Source: three-view drawing plus pictorial views. Frame: mm from the lowest corner of the part. Give positions to 0.01 mm unless a question says otherwise; leave off trailing zeros. Write each loop counter-clockwise with the first axis right and the second up, starting at its lowest first coordinate (ties: lowest second). Pieces come first, ordered by that corner, then holes.
Q1. Cut plane C-C on x = 216. Return the cut outline in (y, z), plus the area to 3 significant figures.
Q2. Cut plane B-B on y = 136.5. Return the cut outline in (x, z), plus the area to 3 significant figures.
Q3. Draft query along Y for the marked faces 1 and 2. Return one class per face: pulls with the +Y half, pulls with the -Y half, needs draft (parallel to the pull), parting line crosses it, or undercut.
Q4. Cut plane D-D on y = 228. Return the cut outline in (x, z), plus the area to 3 significant figures.
Q5. Cut plane A-A on z = 136.5. Return the cut outline in (x, y).
Q6. Pin query (flat end, axial travel): pin 1 (2 mm diameter, centred on x = 117, z = 224.5, fed in from +Y); pin 2 (8 mm diameter, centred on x = 319.5, z = 57, fed in from -Y); pin 3 (8 mm diameter, centred on x = 178.5, z = 287, fed in from +Y). Return the tip coordinate at first contact, or that it passes through.
Q7. Line query: L1, parallel to Z at x = 233, y = 136; L2, parallel to Y at x = 162, z = 143; L3, parallel to Y at x = 216, z = 288.5. Output: solid intervals per line, ascending.
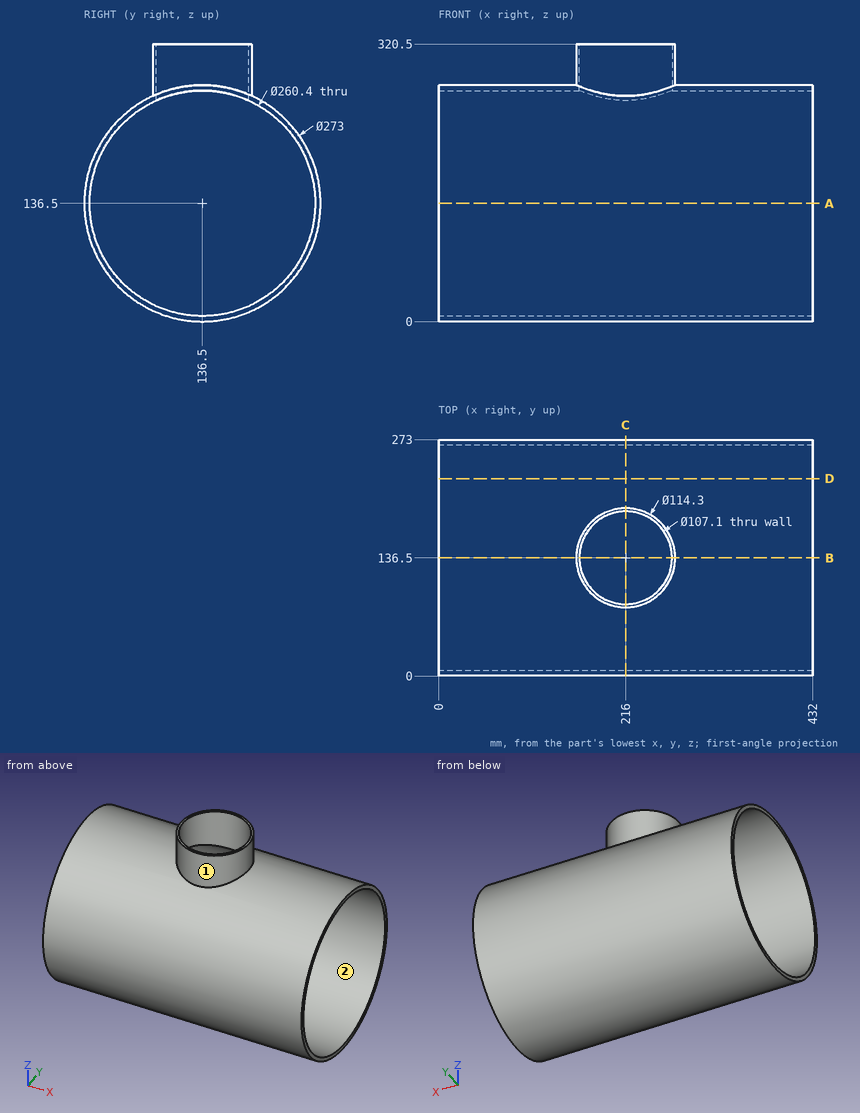
Data:
1. outline: (79.35, 260.46) arc R136.5 ccw (long way) to (193.65, 260.46) - (193.65, 320.5) - (190.05, 320.5) - (190.05, 255.18) arc R130.2 cw (long way) to (82.95, 255.18) - (82.95, 320.5) - (79.35, 320.5) - close
1. area: 5,010 mm2
2. outline: (0, 0) - (432, 0) - (432, 6.3) - (0, 6.3) - close; (0, 266.7) - (162.45, 266.7) - (162.45, 320.5) - (158.85, 320.5) - (158.85, 273) - (0, 273) - close; (269.55, 266.7) - (432, 266.7) - (432, 273) - (273.15, 273) - (273.15, 320.5) - (269.55, 320.5) - close
2. area: 5,110 mm2
3. face 1: parting line crosses it
3. face 2: undercut
4. outline: (0, 35.21) - (432, 35.21) - (432, 43.87) - (0, 43.87) - close; (0, 229.13) - (432, 229.13) - (432, 237.79) - (0, 237.79) - close
4. area: 7,490 mm2
5. outline: (0, 0) - (432, 0) - (432, 6.3) - (0, 6.3) - close; (0, 266.7) - (432, 266.7) - (432, 273) - (0, 273) - close
6. pin 1: stops at y = 241.68
6. pin 2: stops at y = 22.78
6. pin 3: stops at y = 182.8
7. L1: z = 0 to 6.3
7. L2: y = 0.15 to 6.46, 266.54 to 272.85
7. L3: y = 79.35 to 82.95, 190.05 to 193.65
